Geometry check sheet. Reference: the model listing, model coordinates, mm. A direction names the side the tool comes from. Coordinates: 2 decimals unless noted, no trailing zeros. Loops run counter-clockwise (first coordinate to the right, second up) from the corner with the lowest first, then second, coordinate; pieces in that order, holes last. Notation, with made-up numbers: (-17.75, 66.25) -> (3.25, 66.25) arc R17 cw to (3.25, 75.25) -> close; hole circle Ø7 at (8, 2.25). An arc over 180 degrees is marked (long way). Answer as a JSON object with one key per item and string values.
from build123d import *

# Parameters (mm, degrees)
ODGI_CIE_START         = -275
ODGI_CIE_BAZOWE1_DEPTH = 550
ZAOKR_GLENIE1_R        = 25


# Read off the part's stored shape, not the designer's step: Odgięcie bazowe1
with BuildPart() as part:
    # Odgięcie bazowe1 outline → Odgięcie bazowe1 (new body)
    with BuildSketch(Plane(origin=(0, 0, 0), x_dir=(0, 0, -1), z_dir=(1, 0, 0)).offset(ODGI_CIE_START)):
        with BuildLine():
            ThreePointArc((0.974954747, 7.940369213), (-64.137664757, -12.277636548), (-92.140200755, -74.440961373))
            Line((-92.140200755, -74.440961373), (-84.140200755, -74.440961373))
            ThreePointArc((-84.140200755, -74.440961373), (-58.836704372, -18.269282314), (0, 0))
            Line((0, 0), (397.018460657, -48.747737362))
            ThreePointArc((397.018460657, -48.747737362), (453.562640464, -39.116973792), (495.513304801, 0))
            ThreePointArc((495.513304801, 0), (648.639105254, 365.128945319), (700.894657745, 757.603167031))
            Line((700.894657745, 757.603167031), (692.894657745, 757.603167031))
            ThreePointArc((692.894657745, 757.603167031), (640.917801534, 367.222141168), (488.608672016, 4.040550224))
            ThreePointArc((488.608672016, 4.040550224), (450.014060826, -31.947065665), (397.993415404, -40.807368149))
            Line((397.993415404, -40.807368149), (0.974954747, 7.940369213))
        make_face()
    extrude(amount=ODGI_CIE_BAZOWE1_DEPTH)

    # Zaokrąglenie1
    zaokr_glenie1_edges = [part.edges().sort_by_distance(p)[0] for p in [
        (-275, -74.440961373, 88.140200755),
        (275, 757.603167031, -696.894657745),
        (275, -74.440961373, 88.140200755),
        (-275, 757.603167031, -696.894657745),
    ]]
    fillet(zaokr_glenie1_edges, radius=ZAOKR_GLENIE1_R)


solid = part.part
1. Depth check by flat-ended pin: P1, Ø2, axis at x = -175, z = -383, coming from the +Y side; P2, Ø3, axis at x = 213.5, y = 161, coming from the -Z side; P3, Ø1.5, axis at x = 25.5, z = -485.5, coming from the +Y side. Enter the tip coordinate at first touch or a pass-through.
Evaluation:
{"P1": "stops at y = -38.84", "P2": "stops at z = -577.79", "P3": "stops at y = 0.23"}
2. Section check B-B, the plane y = 355. Record the boundary of the cut face in (x, z), then the cut area to 3 significant figures.
Evaluation:
{"outline": "(-275, -645.86) -> (275, -645.86) -> (275, -637.55) -> (-275, -637.55) -> close", "area": "4,570 mm^2"}
3. Tool access check on faces 1 (the face through (-3.85, -16.775, -202.263)), 2 (the face through (-3.85, -24.033, -195.73)), 3 (the face through (-267.482, 750.474, -696.732)). Record the directions out of +Z, -Z, +X, -X, +Y, -Y that give a thin tool (end or side, any length) a straight path to the whole face; none if there is none.
Evaluation:
{"face 1": "+X, -X, +Y", "face 2": "+X, -X, -Y", "face 3": "+Z, -Z, -X, +Y"}
4. Section check C-C, the plane z = 32. Record the boundary of the cut face in (x, y), then the cut area to 3 significant figures.
Evaluation:
{"outline": "(-275, -3.01) -> (275, -3.01) -> (275, 5.35) -> (-275, 5.35) -> close", "area": "4,600 mm^2"}
5. Mould release check, pull along Z, two halves, no side actions. Record for faces 4 (the face through (-3.85, 359.766, -647.175)), 5 (the face through (-3.85, -18.862, 59.499)), 6 (the face through (275, -33.2, -333.6)): released by +Z, released by -Z, zero draft, split by the parting line, or undercut.
Evaluation:
{"face 4": "released by -Z", "face 5": "undercut", "face 6": "zero draft"}
6. Section check A-A, the plane x = 0.5. Record the boundary of the cut face in (y, z).
Evaluation:
{"outline": "(-74.44, 84.14) arc R75 cw to (0, 0) -> (-48.75, -397.02) arc R100 ccw to (0, -495.51) arc R1500 ccw to (757.6, -700.89) -> (757.6, -692.89) arc R1492 cw to (4.04, -488.61) arc R92 cw to (-40.81, -397.99) -> (7.94, -0.97) arc R83 ccw to (-74.44, 92.14) -> close"}
7. Thickness scan on probe 1 along Y at (x, z) = (-191, -407.5); probe 2 along Z at (x, y) = (251, 182); probe 3 along Z at (x, y) = (42, 531.5). Record the ranges inside material, lowest first. Write a range as from..to.
Evaluation:
{"probe 1": "y = -49.48..-41.48", "probe 2": "z = -586.06..-577.39", "probe 3": "z = -683.76..-675.66"}
